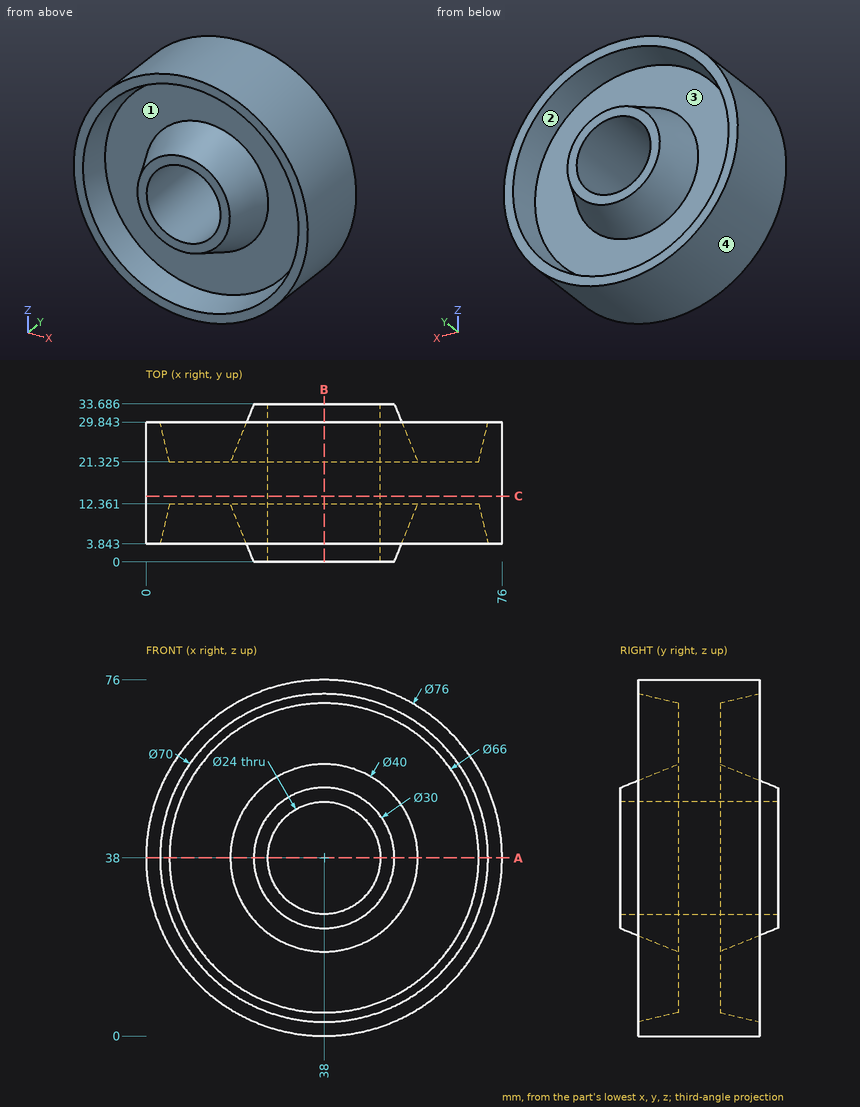
The drawing under review shows one solid part. Ordinate dimensions are in mm from its lowest x, y, z. A direction names the side the tool comes from. Coordinates: 2 decimals unless noted, no trailing zeros. Write each loop counter-clockwise with the first axis right and the second up, starting at its lowest first coordinate (ties: lowest second). Pieces come first, ordered by that corner, then holes. Notation, with made-up numbers: (77, 7) - (121, 7) arc R15 cw to (121, 16) - close; hole circle Ø11 at (80, 59). An arc over 180 degrees is marked (long way). Answer in a Markdown table with one row per item. Add a question column.
Q1. Tool access review of the marked faces 1 and 2: name each direction out of +Z, -Z, +X, -X, +Y, -Y from which nothing blocks a thin tool from reaching the whole face with its end or side.
Q2. We need section A-A, the plane z = 38. State the section outline as (x, y) points (1 decimal).
Q3. For P1, Ø5, axis at y = 13.5, z = 13.5, coming from the +X side (1 decimal); P2, Ø1, axis at x = 20, y = 5, coming from the +Z side; P3, Ø1, axis at x = 26.5, y = 7, coming from the -Z side, all flat-tipped, find the tip position at first contact; note any pin that passes through.
Q4. Draft analysis for pull direction X (two halves, no side actions). For the marked faces 3 and 4, state which applies: +X half, -X half, draft (parallel to the pull), parting line (faces both ways), or undercut.
Q5. We need section C-C, the plane y = 14. State the section outline as (x, z) points.
Q6. For probe 1 along Z at (x, y) = (24.5, 11.5) (1 decimal); probe 2 along X at (y, z) = (15, 38); probe 3 along X at (y, z) = (9, 33), list the stretches that pass through material, from the lowest coordinate up.
Q7. We need section B-B, the plane x = 38. State the section outline as (y, z) points (1 decimal).
Answer list:
| question | item | result |
|---|---|---|
| 1 | face 1 | -Y |
| 1 | face 2 | +Y |
| 2 | outline | (0, 3.8) - (3, 3.8) - (5, 12.4) - (18, 12.4) - (23, 0) - (26, 0) - (26, 33.7) - (23, 33.7) - (18, 21.3) - (5, 21.3) - (3, 29.8) - (0, 29.8) - close; (50, 0) - (53, 0) - (58, 12.4) - (71, 12.4) - (73, 3.8) - (76, 3.8) - (76, 29.8) - (73, 29.8) - (71, 21.3) - (58, 21.3) - (53, 33.7) - (50, 33.7) - close |
| 3 | P1 | stops at x = 69 |
| 3 | P2 | stops at z = 71.73 |
| 3 | P3 | stops at z = 1.63 |
| 4 | face 3 | undercut |
| 4 | face 4 | parting line |
| 5 | outline | circle Ø76 at (38, 38); hole circle Ø24 at (38, 38) |
| 6 | probe 1 | z = 2.5 to 7.7, 23.7 to 52.3, 68.3 to 73.5 |
| 6 | probe 2 | x = 0 to 26, 50 to 76 |
| 6 | probe 3 | x = 0.33 to 4.58, 20.04 to 27.09, 48.91 to 55.96, 71.42 to 75.67 |
| 7 | outline | (0, 23) - (12.4, 18) - (12.4, 5) - (3.8, 3) - (3.8, 0) - (29.8, 0) - (29.8, 3) - (21.3, 5) - (21.3, 18) - (33.7, 23) - (33.7, 26) - (0, 26) - close; (0, 50) - (33.7, 50) - (33.7, 53) - (21.3, 58) - (21.3, 71) - (29.8, 73) - (29.8, 76) - (3.8, 76) - (3.8, 73) - (12.4, 71) - (12.4, 58) - (0, 53) - close |
